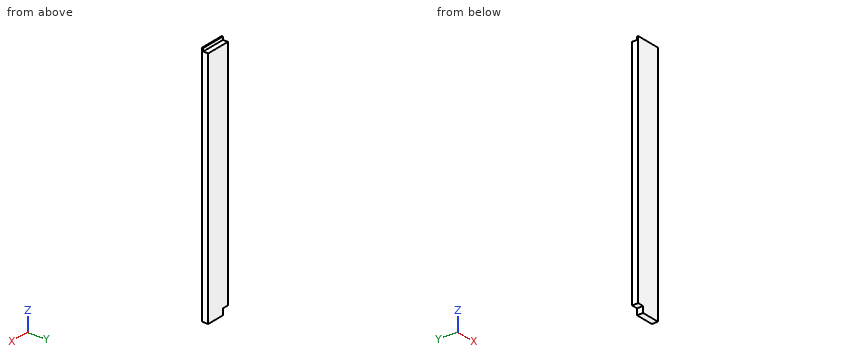
```python
from build123d import *

# Parameters (mm, degrees)
BOSS_EXTRUDE1_DEPTH = 501.65
SKETCH2_W           = 50.8
SKETCH2_H           = 6.35
CUT_EXTRUDE1_DEPTH  = 10.3378
SKETCH3_W           = 12.7
SKETCH3_H           = 12.7
CUT_EXTRUDE2_DEPTH  = 13.7


with BuildPart() as part:
    # Sketch1 → Boss-Extrude1 (new body)
    with BuildSketch(Plane.XY):
        Polygon((0, 12.7), (0, 6.35), (0, 0), (12.7, 0), (50.8, 0), (50.8, 12.7), align=None)
    extrude(amount=BOSS_EXTRUDE1_DEPTH)

    # Sketch2 → Cut-Extrude1 (cut)
    with BuildSketch(Plane.XZ.offset(-12.7)):
        with Locations((25.4, 498.475)):
            Rectangle(SKETCH2_W, SKETCH2_H)
    extrude(amount=CUT_EXTRUDE1_DEPTH, mode=Mode.SUBTRACT)

    # Sketch3 → Cut-Extrude2 (cut, through all)
    with BuildSketch(Plane(origin=(0, 12.7, 0), x_dir=(1, 0, 0), z_dir=(0, 1, 0))):
        with Locations((6.35, -6.35)):
            Rectangle(SKETCH3_W, SKETCH3_H)
    extrude(amount=-CUT_EXTRUDE2_DEPTH, mode=Mode.SUBTRACT)


solid = part.part
```
CAD build for the part. Positions are in the model's coordinates, mm. Give positions to 0.01 mm unless a question says otherwise; leave off trailing zeros. Loops run counter-clockwise (first coordinate to the right, second up) from the corner with the lowest first, then second, coordinate; pieces in that order, holes last. Notation, with made-up numbers: (-24, 26) - (-7, 26) arc R24 ccw to (-7, 63) - close; hole circle Ø11 at (73.5, 40.25). An arc over 180 degrees is marked (long way). Put each result on its own line as item: value.
Q1. Slice it at A-A (y = 10.25). Give the cut face in (x, z).
Filled in:
outline: (0, 12.7) - (12.7, 12.7) - (12.7, 0) - (50.8, 0) - (50.8, 495.3) - (0, 495.3) - close
Q2. Slice it at B-B (x = 8.5). Give the cut face in (y, z), plus the area to 3 significant figures.
Filled in:
outline: (0, 12.7) - (12.7, 12.7) - (12.7, 495.3) - (2.36, 495.3) - (2.36, 501.65) - (0, 501.65) - close
area: 6,140 mm²
Q3. Flat gauge pin, fed straight in: pin 1 (2 mm diameter, centred on x = 17.5, y = 8.5, fed in from +Z). Where does the tip first touch, or does it go through?
Filled in:
pin 1: stops at z = 495.3
Q4. Probe line 1 along Z through (x, y) = (48.5, 7); line 2 along Z through (x, y) = (8, 7.75). List the from-to ranges inside material, lowest first.
Filled in:
line 1: z = 0 to 495.3
line 2: z = 12.7 to 495.3
